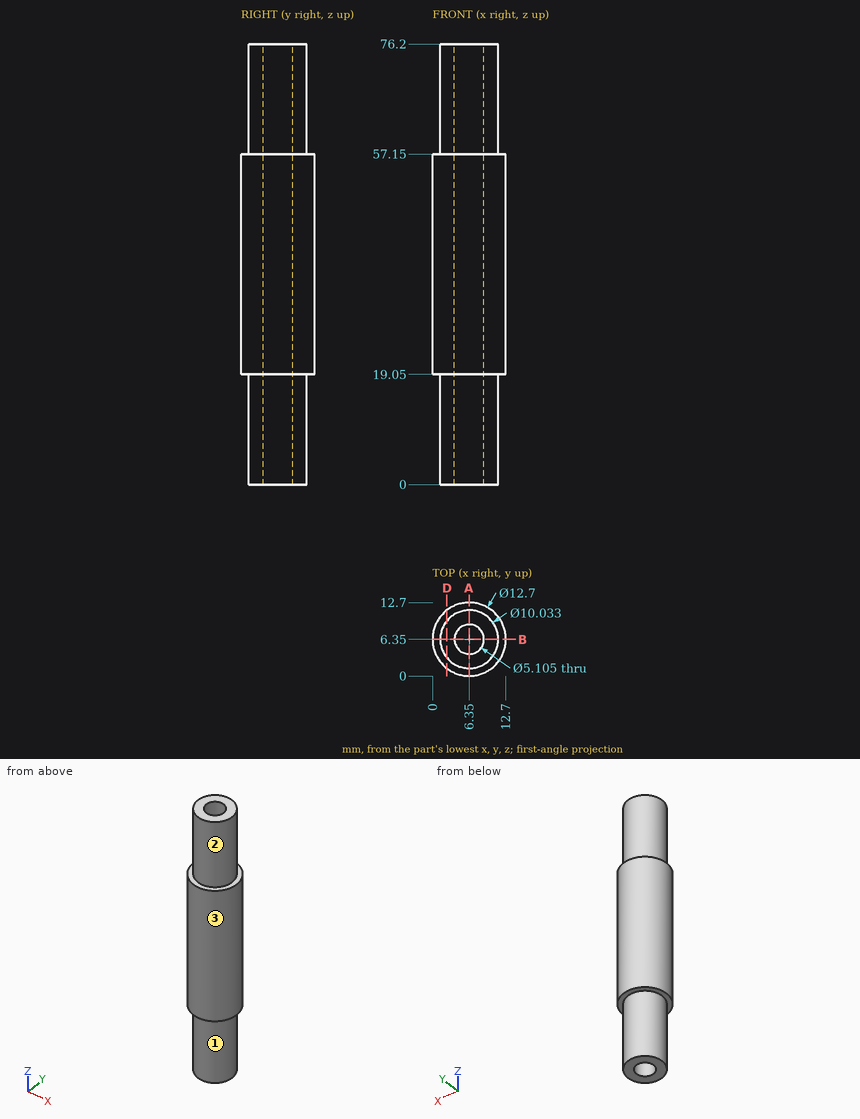
The figure shows three views and two pictorial views of one solid part (mm, origin at its lowest corner). Answer the questions. A direction names the side the tool comes from. Round coordinates to 2 decimals unless told otherwise and drop trailing zeros. Loops run counter-clockwise (first coordinate to the right, second up) from the corner with the lowest first, then second, coordinate; pieces in that order, holes last. Notation, with made-up numbers: (20.5, 55.25) - (75.5, 55.25) arc R16 cw to (75.5, 70.25) - close; hole circle Ø9 at (88, 86.5). An arc over 180 degrees is marked (long way). Use one line per item in the form item = value. Start each with the question number.
(1) Consider line 1 (Y direction, x = 6.35, z = 21.5); line 2 (Z direction, x = 2.5, y = 9.75); line 3 (Y direction, x = 4.5, z = 70) (1 decimal). Determine where each line is inside the solid, lowest interval first.
(2) Find section D-D on x = 2.5. Determine the outline of the cut face in (y, z), and give its area (3 significant figures).
(3) Find section A-A on x = 6.35. Determine the outline of the cut face in (y, z), and give its area (3 significant figures).
(4) Flat-ended cylindrical pins translate along their axes: P1, Ø2, axis at y = 5.5, z = 62, coming from the -X side; P2, Ø5, axis at y = 1.5, z = 29.5, coming from the +X side; P3, Ø3, axis at x = 9.5, z = 35.5, coming from the -Y side. Find the tip coordinate at first contact, or state that the pin passes through.
(5) Which of the six approach directions +Z, -Z, +X, -X, +Y, -Y give full straight-line access (tool end or side, diameter ignored) to the marked faces 1, 2 and 3?
Answer list:
q1.line_1 = 0 to 3.8, 8.9 to 12.7
q1.line_2 = 19.05 to 57.15
q1.line_3 = 1.7 to 4.6, 8.1 to 11
q2.outline = (1.3, 19.05) - (3.13, 19.05) - (3.13, 0) - (9.57, 0) - (9.57, 19.05) - (11.4, 19.05) - (11.4, 57.15) - (9.57, 57.15) - (9.57, 76.2) - (3.13, 76.2) - (3.13, 57.15) - (1.3, 57.15) - close
q2.area = 630 mm^2
q3.outline = (0, 19.05) - (1.33, 19.05) - (1.33, 0) - (3.8, 0) - (3.8, 76.2) - (1.33, 76.2) - (1.33, 57.15) - (0, 57.15) - close; (8.9, 0) - (11.37, 0) - (11.37, 19.05) - (12.7, 19.05) - (12.7, 57.15) - (11.37, 57.15) - (11.37, 76.2) - (8.9, 76.2) - close
q3.area = 477 mm^2
q4.P1 = 1.33
q4.P2 = 12.25
q4.P3 = 0.22
q5.face_1 = -Z
q5.face_2 = +Z
q5.face_3 = +Z, -Z
